Geometry: see drawing. Coordinates: mm, zero at the bounding-box minimum. A direction names the side the tool comes from. Coordinates: 2 decimals unless noted, no trailing zeros. Order: outer loops, then holes, each group sorted by start corner. A loop starts at its lowest first (then second) coordinate and runs counter-clockwise, first axis right, second up.
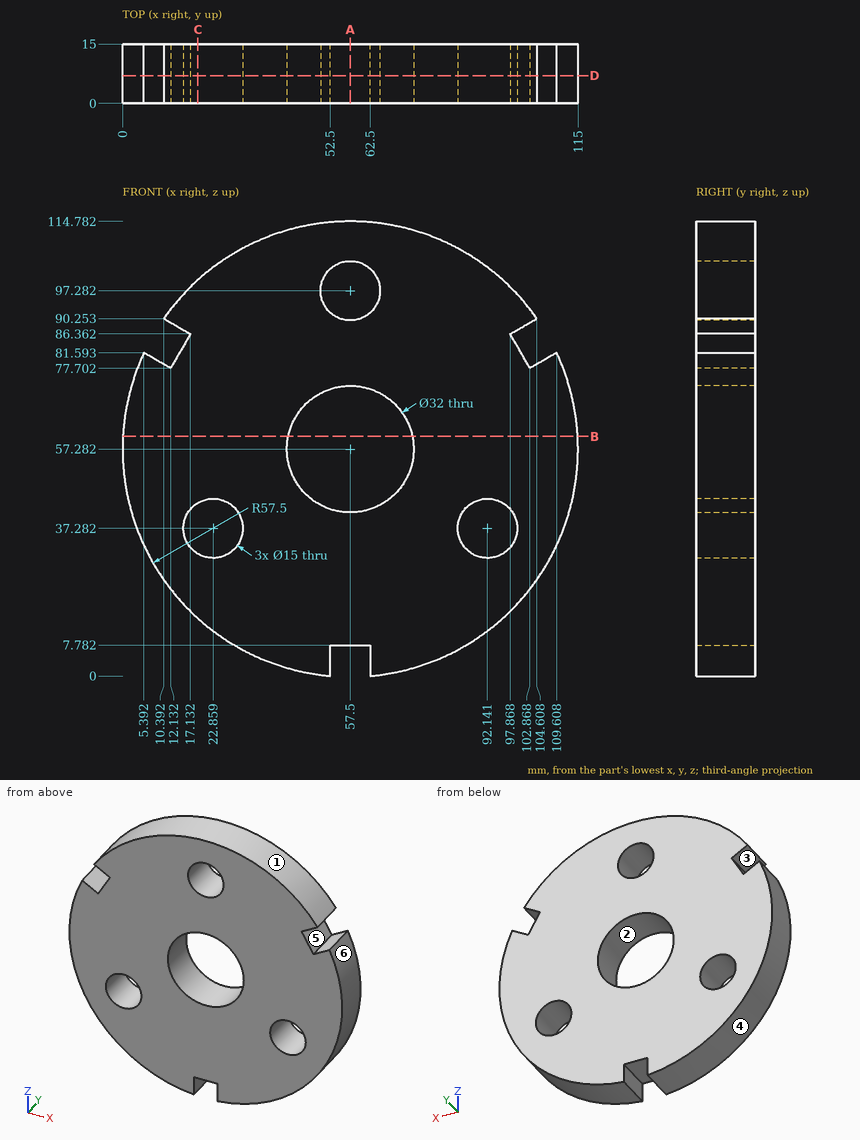
Item 1: Cut plane C-C on x = 19. Return loops of the section in (y, z).
Response values:
outline: (0, 14.57) - (15, 14.57) - (15, 30.85) - (0, 30.85) - close; (0, 43.71) - (15, 43.71) - (15, 99.99) - (0, 99.99) - close
Item 2: Draft query along Z for the marked faces 1, 2, 3 and 4. Return one class per face: pulls with the +Z half, pulls with the -Z half, needs draft (parallel to the pull), parting line crosses it, or undercut.
Response values:
face 1: pulls with the +Z half
face 2: undercut
face 3: undercut
face 4: parting line crosses it
Item 3: Cut plane B-B on z = 60.5. Return loops of the section in (x, y), then the cut area to 3 significant figures.
Response values:
outline: (0.09, 0) - (41.83, 0) - (41.83, 15) - (0.09, 15) - close; (73.17, 0) - (114.91, 0) - (114.91, 15) - (73.17, 15) - close
area: 1,250 mm2
Item 4: Ray query, probe 1 along Z at (x, y) = (57.5, 8); probe 2 along Z at (x, y) = (54.5, 13.25) (1 decimal); probe 3 along X at (y, z) = (13.25, 30.5) (1 decimal). Return the intervals inside material, ascending.
Response values:
probe 1: z = 7.78 to 41.28, 73.28 to 89.78, 104.78 to 114.78
probe 2: z = 7.8 to 41.6, 73 to 90.4, 104.2 to 114.7
probe 3: x = 6.6 to 19.7, 26.1 to 88.9, 95.3 to 108.4
Item 5: Pin query (flat end, axial travel): pin 1 Ø4 at (y, z) = (10.5, 4) entering from +X (1 decimal); pin 2 Ø4 at (y, z) = (5.5, 3.5) entering from -X (1 decimal); pin 3 Ø3 at (y, z) = (6, 74) entering from +X. Return the tip coordinate at first contact, or that it passes through.
Response values:
pin 1: stops at x = 83.5
pin 2: stops at x = 32.5
pin 3: stops at x = 112.95
Item 6: Cut plane D-D on y = 7. Return loops of the section in (x, z).
Response values:
outline: (5.39, 81.59) arc R57.5 ccw to (52.5, 0) - (52.5, 7.78) - (62.5, 7.78) - (62.5, 0) arc R57.5 ccw to (109.61, 81.59) - (102.87, 77.7) - (97.87, 86.36) - (104.61, 90.25) arc R57.5 ccw to (10.39, 90.25) - (17.13, 86.36) - (12.13, 77.7) - close; hole circle Ø15 at (22.86, 37.28); hole circle Ø32 at (57.5, 57.28); hole circle Ø15 at (57.5, 97.28); hole circle Ø15 at (92.14, 37.28)
Item 7: Cut plane A-A on x = 57.5. Return loops of the section in (y, z), then the cut area to 3 significant figures.
Response values:
outline: (0, 7.78) - (15, 7.78) - (15, 41.28) - (0, 41.28) - close; (0, 73.28) - (15, 73.28) - (15, 89.78) - (0, 89.78) - close; (0, 104.78) - (15, 104.78) - (15, 114.78) - (0, 114.78) - close
area: 900 mm2
Item 8: Access query for the marked faces 5 and 6. Directions: +Z, -Z, +X, -X, +Y, -Y. A direction counts if a zero-diameter tool reaches every point of the face in a straight line with its end or side. Return the directions, or none.
Response values:
face 5: +Y, -Y
face 6: +X, +Y, -Y
